```python
from build123d import *

# Parameters (mm, degrees)
SKETCH_3_R      = 3.4
EXTRUDE_1_DEPTH = 2488


with BuildPart() as part:
    # 草图3 → 凸台-拉伸1 (new body)
    with BuildSketch(Plane(origin=(0, 0, 0), x_dir=(1, 0, 0), z_dir=(0, 1, 0))):
        with BuildLine():
            Line((-15, -12.5), (-15, -5.4))
            ThreePointArc((-15, -5.4), (-14.941421356, -5.258578644), (-14.8, -5.2))
            Line((-14.8, -5.2), (-14.4, -5.2))
            ThreePointArc((-14.4, -5.2), (-14.258578644, -5.141421356), (-14.2, -5))
            Line((-14.2, -5), (-14.2, -4.3))
            ThreePointArc((-14.2, -4.3), (-14.141421356, -4.158578644), (-14, -4.1))
            Line((-14, -4.1), (-13.2, -4.1))
            Line((-13.2, -4.1), (-13.2, -8.25))
            Line((-13.2, -8.25), (-9.522792206, -8.25))
            Line((-9.522792206, -8.25), (-5.8, -4.527207794))
            Line((-5.8, -4.527207794), (-5.8, 4.527207794))
            Line((-5.8, 4.527207794), (-9.522792206, 8.25))
            Line((-9.522792206, 8.25), (-13.2, 8.25))
            Line((-13.2, 8.25), (-13.2, 4.1))
            Line((-13.2, 4.1), (-14, 4.1))
            ThreePointArc((-14, 4.1), (-14.141421356, 4.158578644), (-14.2, 4.3))
            Line((-14.2, 4.3), (-14.2, 5))
            ThreePointArc((-14.2, 5), (-14.258578644, 5.141421356), (-14.4, 5.2))
            Line((-14.4, 5.2), (-14.8, 5.2))
            ThreePointArc((-14.8, 5.2), (-14.941421356, 5.258578644), (-15, 5.4))
            Line((-15, 5.4), (-15, 12.5))
            ThreePointArc((-15, 12.5), (-14.267766953, 14.267766953), (-12.5, 15))
            Line((-12.5, 15), (-5.4, 15))
            ThreePointArc((-5.4, 15), (-5.258578644, 14.941421356), (-5.2, 14.8))
            Line((-5.2, 14.8), (-5.2, 14.4))
            ThreePointArc((-5.2, 14.4), (-5.141421356, 14.258578644), (-5, 14.2))
            Line((-5, 14.2), (-4.3, 14.2))
            ThreePointArc((-4.3, 14.2), (-4.158578644, 14.141421356), (-4.1, 14))
            Line((-4.1, 14), (-4.1, 13.2))
            Line((-4.1, 13.2), (-8.25, 13.2))
            Line((-8.25, 13.2), (-8.25, 9.522792206))
            Line((-8.25, 9.522792206), (-4.527207794, 5.8))
            Line((-4.527207794, 5.8), (4.527207794, 5.8))
            Line((4.527207794, 5.8), (8.25, 9.522792206))
            Line((8.25, 9.522792206), (8.25, 13.2))
            Line((8.25, 13.2), (4.1, 13.2))
            Line((4.1, 13.2), (4.1, 14))
            ThreePointArc((4.1, 14), (4.158578644, 14.141421356), (4.3, 14.2))
            Line((4.3, 14.2), (5, 14.2))
            ThreePointArc((5, 14.2), (5.141421356, 14.258578644), (5.2, 14.4))
            Line((5.2, 14.4), (5.2, 14.8))
            ThreePointArc((5.2, 14.8), (5.258578644, 14.941421356), (5.4, 15))
            Line((5.4, 15), (12.5, 15))
            ThreePointArc((12.5, 15), (14.267766953, 14.267766953), (15, 12.5))
            Line((15, 12.5), (15, 5.4))
            ThreePointArc((15, 5.4), (14.941421356, 5.258578644), (14.8, 5.2))
            Line((14.8, 5.2), (14.4, 5.2))
            ThreePointArc((14.4, 5.2), (14.258578644, 5.141421356), (14.2, 5))
            Line((14.2, 5), (14.2, 4.3))
            ThreePointArc((14.2, 4.3), (14.141421356, 4.158578644), (14, 4.1))
            Line((14, 4.1), (13.2, 4.1))
            Line((13.2, 4.1), (13.2, 8.25))
            Line((13.2, 8.25), (9.522792206, 8.25))
            Line((9.522792206, 8.25), (5.8, 4.527207794))
            Line((5.8, 4.527207794), (5.8, -4.527207794))
            Line((5.8, -4.527207794), (9.522792206, -8.25))
            Line((9.522792206, -8.25), (13.2, -8.25))
            Line((13.2, -8.25), (13.2, -4.1))
            Line((13.2, -4.1), (14, -4.1))
            ThreePointArc((14, -4.1), (14.141421356, -4.158578644), (14.2, -4.3))
            Line((14.2, -4.3), (14.2, -5))
            ThreePointArc((14.2, -5), (14.258578644, -5.141421356), (14.4, -5.2))
            Line((14.4, -5.2), (14.8, -5.2))
            ThreePointArc((14.8, -5.2), (14.941421356, -5.258578644), (15, -5.4))
            Line((15, -5.4), (15, -12.5))
            ThreePointArc((15, -12.5), (14.267766953, -14.267766953), (12.5, -15))
            Line((12.5, -15), (5.4, -15))
            ThreePointArc((5.4, -15), (5.258578644, -14.941421356), (5.2, -14.8))
            Line((5.2, -14.8), (5.2, -14.4))
            ThreePointArc((5.2, -14.4), (5.141421356, -14.258578644), (5, -14.2))
            Line((5, -14.2), (4.3, -14.2))
            ThreePointArc((4.3, -14.2), (4.158578644, -14.141421356), (4.1, -14))
            Line((4.1, -14), (4.1, -13.2))
            Line((4.1, -13.2), (8.25, -13.2))
            Line((8.25, -13.2), (8.25, -9.522792206))
            Line((8.25, -9.522792206), (4.527207794, -5.8))
            Line((4.527207794, -5.8), (-4.527207794, -5.8))
            Line((-4.527207794, -5.8), (-8.25, -9.522792206))
            Line((-8.25, -9.522792206), (-8.25, -13.2))
            Line((-8.25, -13.2), (-4.1, -13.2))
            Line((-4.1, -13.2), (-4.1, -14))
            ThreePointArc((-4.1, -14), (-4.158578644, -14.141421356), (-4.3, -14.2))
            Line((-4.3, -14.2), (-5, -14.2))
            ThreePointArc((-5, -14.2), (-5.141421356, -14.258578644), (-5.2, -14.4))
            Line((-5.2, -14.4), (-5.2, -14.8))
            ThreePointArc((-5.2, -14.8), (-5.258578644, -14.941421356), (-5.4, -15))
            Line((-5.4, -15), (-12.5, -15))
            ThreePointArc((-12.5, -15), (-14.267766953, -14.267766953), (-15, -12.5))
        make_face()
        Circle(SKETCH_3_R, mode=Mode.SUBTRACT)
        with BuildLine():
            Line((-13.2, -12.2), (-13.2, -11.05))
            ThreePointArc((-13.2, -11.05), (-12.907106781, -10.342893219), (-12.2, -10.05))
            Line((-12.2, -10.05), (-11.05, -10.05))
            ThreePointArc((-11.05, -10.05), (-10.342893219, -10.342893219), (-10.05, -11.05))
            Line((-10.05, -11.05), (-10.05, -12.2))
            ThreePointArc((-10.05, -12.2), (-10.342893219, -12.907106781), (-11.05, -13.2))
            Line((-11.05, -13.2), (-12.2, -13.2))
            ThreePointArc((-12.2, -13.2), (-12.907106781, -12.907106781), (-13.2, -12.2))
        make_face(mode=Mode.SUBTRACT)
        with BuildLine():
            Line((-10.05, 12.2), (-10.05, 11.05))
            ThreePointArc((-10.05, 11.05), (-10.342893219, 10.342893219), (-11.05, 10.05))
            Line((-11.05, 10.05), (-12.2, 10.05))
            ThreePointArc((-12.2, 10.05), (-12.907106781, 10.342893219), (-13.2, 11.05))
            Line((-13.2, 11.05), (-13.2, 12.2))
            ThreePointArc((-13.2, 12.2), (-12.907106781, 12.907106781), (-12.2, 13.2))
            Line((-12.2, 13.2), (-11.05, 13.2))
            ThreePointArc((-11.05, 13.2), (-10.342893219, 12.907106781), (-10.05, 12.2))
        make_face(mode=Mode.SUBTRACT)
        with BuildLine():
            Line((13.2, 12.2), (13.2, 11.05))
            ThreePointArc((13.2, 11.05), (12.907106781, 10.342893219), (12.2, 10.05))
            Line((12.2, 10.05), (11.05, 10.05))
            ThreePointArc((11.05, 10.05), (10.342893219, 10.342893219), (10.05, 11.05))
            Line((10.05, 11.05), (10.05, 12.2))
            ThreePointArc((10.05, 12.2), (10.342893219, 12.907106781), (11.05, 13.2))
            Line((11.05, 13.2), (12.2, 13.2))
            ThreePointArc((12.2, 13.2), (12.907106781, 12.907106781), (13.2, 12.2))
        make_face(mode=Mode.SUBTRACT)
        with BuildLine():
            Line((10.05, -12.2), (10.05, -11.05))
            ThreePointArc((10.05, -11.05), (10.342893219, -10.342893219), (11.05, -10.05))
            Line((11.05, -10.05), (12.2, -10.05))
            ThreePointArc((12.2, -10.05), (12.907106781, -10.342893219), (13.2, -11.05))
            Line((13.2, -11.05), (13.2, -12.2))
            ThreePointArc((13.2, -12.2), (12.907106781, -12.907106781), (12.2, -13.2))
            Line((12.2, -13.2), (11.05, -13.2))
            ThreePointArc((11.05, -13.2), (10.342893219, -12.907106781), (10.05, -12.2))
        make_face(mode=Mode.SUBTRACT)
    extrude(amount=EXTRUDE_1_DEPTH)


solid = part.part
```
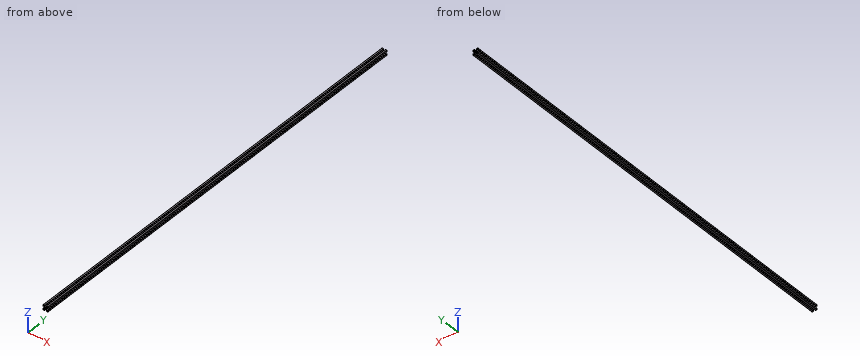
The model under review builds one solid part; all positions refer to its coordinate system, in mm. Round coordinates to 2 decimals unless told otherwise and drop trailing zeros. Use one line per item in the form item = value.
Q1. For line 1 (Z direction, x = 6.5, y = 1283); line 2 (X direction, y = 1389.5, z = -10.25); line 3 (X direction, y = 766.5, z = 11), list the stretches that pass through material, from the lowest coordinate up. Write a range as [from, to].
Answer key:
line_1 = [-15, -13.2], [-7.77, -5.23], [5.23, 7.77], [13.2, 15]
line_2 = [-15, -12.8], [-10.45, -8.25], [8.25, 10.45], [12.8, 15]
line_3 = [-15, -13.2], [-10.05, -8.25], [8.25, 10.05], [13.2, 15]
Q2. Consider section A-A (y = 359). State how many separate pieces and enclosed holes the cut face has, and give its area (3 significant figures).
Answer key:
separate_pieces = 1
enclosed_holes = 5
area = 323 mm2
Q3. Insertion check: pin 1 Ø8 at (x, y) = (1, 1630.5) entering from -Z; pin 2 Ø6 at (x, z) = (0, 0) entering from +Y. Each pin has a flat end and moves straight along its axis. Give the tip position at first contact, or say it passes through.
Answer key:
pin_1 = -14.2
pin_2 = through
